```python
from build123d import *

# Parameters (mm, degrees)
F0_W     = 20
F0_H     = 11
F1_DEPTH = 20
F2_R     = 2.8
F3_DEPTH = 25
F5_DEPTH = 20
F6_R     = 2.6
F7_DEPTH = 25
F8_SIZE  = 4


# Not quite as in the source:
# - a feature names something its author has since deleted; it is built from what else it names


with BuildPart() as f1:
    # F0 (on Top) → F1 (new body)
    with BuildSketch(Plane.XY):
        with Locations((10, 25.5)):
            Rectangle(F0_W, F0_H)
    extrude(amount=F1_DEPTH)

    # F2 (on face) → F3 (cut)
    with BuildSketch(Plane(origin=(0, 31, 0), x_dir=(-1, 0, 0), z_dir=(0, 1, 0))):
        with Locations((-10, 10)):
            Circle(F2_R)
    extrude(amount=-F3_DEPTH, mode=Mode.SUBTRACT)

    # F4 (on face) → F5 (join, through all)
    with BuildSketch(Plane.XY.offset(20)):
        Polygon((21, 20), (21, 18), (36.3, 18), (36.3, 31), (20, 31), (20, 20), align=None)
    extrude(amount=-F5_DEPTH)

    # F6 (on face) → F7 (cut)
    with BuildSketch(Plane.XZ.offset(-18)):
        with Locations((28.8, 10)):
            Circle(F6_R)
    extrude(amount=-F7_DEPTH, mode=Mode.SUBTRACT)

    # F8
    f8_edges = [f1.edges().sort_by_distance(p)[0] for p in [
        (12.8, 20, 10),
    ]]
    chamfer(f8_edges, length=F8_SIZE)


solid = f1.part
```
The model under review builds one solid part; all positions refer to its coordinate system, in mm. A direction names the side the tool comes from. Coordinates: 2 decimals unless noted, no trailing zeros. Order: outer loops, then holes, each group sorted by start corner. A loop starts at its lowest first (then second) coordinate and runs counter-clockwise, first axis right, second up. Notation, with made-up numbers: (49.5, 24) -> (53.5, 24) arc R16 ccw to (53.5, 42) -> close; hole circle Ø5 at (66.25, 15.5). An arc over 180 degrees is marked (long way). Answer in a Markdown table with one row per item. Add a question column.
Item 1: Clearance check with a flat-ended pin moving along its axis: pin 1 (4 mm diameter, centred on y = 28.5, z = 4.5, fed in from -X). State where the tip first meets the part, or that it passes through.
Item 2: We need section B-B on z = 10. Write out the cut boundary in (x, y).
Item 3: To check wall thickness, follow probe 1 along Z at (x, y) = (28.8, 26.5); probe 2 along X at (y, z) = (25.75, 7.75); probe 3 along Z at (x, y) = (10, 29.75). State the ranges of each line that lie inside material, in increasing order.
Item 4: Machinability: for faces 5 (the flat face through (18, 25, 0)), 6 (the flat face through (10, 20, 17)), which of the approach directions +Z, -Z, +X, -X, +Y, -Y give a long, thin tool a straight path to every point of the face, cutting with its end or side? Answer none if there is none.
Item 5: We need section A-A on x = 28.8. Write out the cut boundary in (y, z).
Item 6: Mouldability with a two-part tool opening along Z and no side actions: class faces 1 (the cylindrical face through (26.737, 24.409, 8.418)), 2 (the conical face through (8.618, 23.806, 7.344)), 3 (the flat face through (21, 19, 10)), 4 (the flat face through (18, 25, 20)) as +Z half, -Z half, draft (parallel to the pull), parting line (faces both ways), or undercut.
Item 7: We need section C-C on y = 22. Write out the cut boundary in (x, z).
Item 8: We need section D-D on x = 10. Write out the cut boundary in (y, z).
Final values:
| question | item | result |
|---|---|---|
| 1 | pin 1 | stops at x = 0 |
| 2 | outline | (0, 20) -> (3.2, 20) -> (7.2, 24) -> (7.2, 31) -> (0, 31) -> close; (12.8, 24) -> (16.8, 20) -> (21, 20) -> (21, 18) -> (26.2, 18) -> (26.2, 31) -> (12.8, 31) -> close; (31.4, 18) -> (36.3, 18) -> (36.3, 31) -> (31.4, 31) -> close |
| 3 | probe 1 | z = 0 to 7.4, 12.6 to 20 |
| 3 | probe 2 | x = 0 to 8.33, 11.67 to 27.5, 30.1 to 36.3 |
| 3 | probe 3 | z = 0 to 7.2, 12.8 to 20 |
| 4 | face 5 | -Z, +X, -X, +Y, -Y |
| 4 | face 6 | +Z, -Z, -X, -Y |
| 5 | outline | (18, 0) -> (31, 0) -> (31, 7.4) -> (18, 7.4) -> close; (18, 12.6) -> (31, 12.6) -> (31, 20) -> (18, 20) -> close |
| 6 | face 1 | undercut |
| 6 | face 2 | undercut |
| 6 | face 3 | draft |
| 6 | face 4 | +Z half |
| 7 | outline | (0, 0) -> (36.3, 0) -> (36.3, 20) -> (0, 20) -> close; hole circle Ø9.6 at (10, 10); hole circle Ø5.2 at (28.8, 10) |
| 8 | outline | (20, 0) -> (31, 0) -> (31, 7.2) -> (24, 7.2) -> (20, 3.2) -> close; (20, 16.8) -> (24, 12.8) -> (31, 12.8) -> (31, 20) -> (20, 20) -> close |
